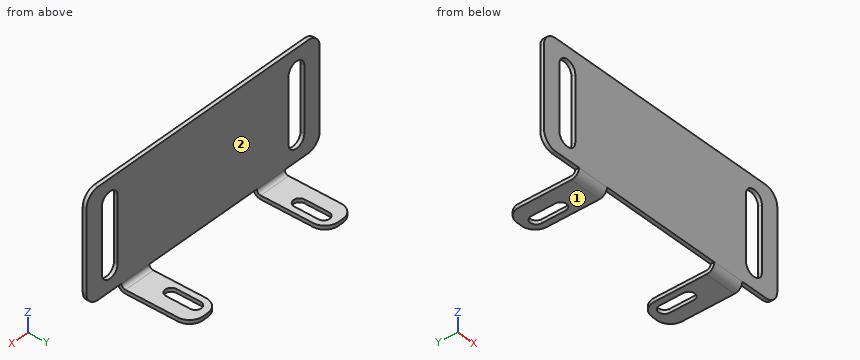
```python
from build123d import *

# Parameters (mm, degrees)
SKETCH1_W             = 50
SKETCH1_H             = 20
BASE_FLANGE1_DEPTH    = 0.7
EDGE_FLANGE1_DEPTH    = 6
CUT_EXTRUDE1_REACH    = 37.405
BREAK_CORNER1_START   = -12
BREAK_CORNER1_DEPTH   = 2
BREAK_CORNER1_START_2 = -2
BREAK_CORNER1_2_DEPTH = 3
CUT_EXTRUDE2_REACH    = 32.41


with BuildPart() as part:
    # Base-Flange1: sheet metal written as solids
    # Sketch1 → Base-Flange1 (new body)
    with BuildSketch(Plane(origin=(0, 0, 0), x_dir=(1, 0, 0), z_dir=(0, 1, 0))):
        Rectangle(SKETCH1_W, SKETCH1_H)
    extrude(amount=-BASE_FLANGE1_DEPTH)

    # Edge-Flange1: sheet metal written as solids
    # Edge-Flange1 section (on a plane across the edge) → Edge-Flange1 (add)
    with BuildSketch(Plane(origin=(17.5, 0, -10.7366), x_dir=(0, 0, 1), z_dir=(-1, 0, 0))):
        with BuildLine():
            Line((-0.7, 0.7366), (-0.7, 13))
            Line((-0.7, 13), (0, 13))
            Line((0, 13), (0, 0.7366))
            ThreePointArc((0, 0.7366), (0.215745145, 0.215745145), (0.7366, 0))
            Line((0.7366, 0), (0.7366, -0.7))
            ThreePointArc((0.7366, -0.7), (-0.279229602, -0.279229602), (-0.7, 0.7366))
        make_face()
    edge_flange1 = extrude(amount=EDGE_FLANGE1_DEPTH)

    # Sketch7 → Cut-Extrude1 (cut, up to next)
    with BuildSketch(Plane(origin=(0, 0, -11.4366), x_dir=(-1, 0, 0), z_dir=(0, 0, -1)), mode=Mode.PRIVATE) as cut_extrude1_sk1:
        with BuildLine():
            Line((-12.65, 10.5), (-12.65, 6))
            ThreePointArc((-12.65, 6), (-13.75, 4.9), (-14.85, 6))
            Line((-14.85, 6), (-14.85, 10.5))
            ThreePointArc((-14.85, 10.5), (-13.75, 11.6), (-12.65, 10.5))
        make_face()
    cut_extrude1_tool1 = extrude(cut_extrude1_sk1.sketch, amount=-CUT_EXTRUDE1_REACH, mode=Mode.PRIVATE) & part.part
    cut_extrude1 = cut_extrude1_tool1.solids().sort_by_distance((13.75, 8.25, -11.4366))[0]
    add(cut_extrude1, mode=Mode.SUBTRACT)

    # Mirror1: Edge-Flange1, Cut-Extrude1 across plane
    add(edge_flange1.mirror(Plane(origin=(0, 0, 0), x_dir=(0, 0, 1), z_dir=(1, 0, 0))))
    add(cut_extrude1.mirror(Plane(origin=(0, 0, 0), x_dir=(0, 0, 1), z_dir=(1, 0, 0))), mode=Mode.SUBTRACT)

    # Break-Corner1: read off the stored shape, not the designer's step
    # Break-Corner1 outline → Break-Corner1 (cut)
    with BuildSketch(Plane.XY.offset(BREAK_CORNER1_START)):
        with BuildLine():
            ThreePointArc((-17.5, 10.5), (-16.767766953, 12.267766953), (-15, 13))
            Line((-15, 13), (-17.5, 13))
            Line((-17.5, 13), (-17.5, 10.5))
        make_face()
        with BuildLine():
            ThreePointArc((-14, 13), (-12.232233047, 12.267766953), (-11.5, 10.5))
            Line((-11.5, 10.5), (-11.5, 13))
            Line((-11.5, 13), (-14, 13))
        make_face()
        with BuildLine():
            ThreePointArc((11.5, 10.5), (12.232233047, 12.267766953), (14, 13))
            Line((14, 13), (11.5, 13))
            Line((11.5, 13), (11.5, 10.5))
        make_face()
        with BuildLine():
            ThreePointArc((15, 13), (16.767766953, 12.267766953), (17.5, 10.5))
            Line((17.5, 10.5), (17.5, 13))
            Line((17.5, 13), (15, 13))
        make_face()
    extrude(amount=BREAK_CORNER1_DEPTH, mode=Mode.SUBTRACT)

    # Break-Corner1 2 outline → Break-Corner1 2 (cut)
    with BuildSketch(Plane(origin=(0, 0, 0), x_dir=(1, 0, 0), z_dir=(0, 1, 0)).offset(BREAK_CORNER1_START_2)):
        with BuildLine():
            ThreePointArc((22.5, 10), (24.267766953, 9.267766953), (25, 7.5))
            Line((25, 7.5), (25, 10))
            Line((25, 10), (22.5, 10))
        make_face()
        with BuildLine():
            Line((-25, 10), (-25, 7.5))
            ThreePointArc((-25, 7.5), (-24.267766953, 9.267766953), (-22.5, 10))
            Line((-22.5, 10), (-25, 10))
        make_face()
        with BuildLine():
            Line((-25, -10), (-22.5, -10))
            ThreePointArc((-22.5, -10), (-24.267766953, -9.267766953), (-25, -7.5))
            Line((-25, -7.5), (-25, -10))
        make_face()
        with BuildLine():
            ThreePointArc((25, -7.5), (24.267766953, -9.267766953), (22.5, -10))
            Line((22.5, -10), (25, -10))
            Line((25, -10), (25, -7.5))
        make_face()
    extrude(amount=BREAK_CORNER1_2_DEPTH, mode=Mode.SUBTRACT)

    # Sketch8 → Cut-Extrude2 (cut, up to next)
    with BuildSketch(Plane(origin=(0, 0, 0), x_dir=(1, 0, 0), z_dir=(0, 1, 0)), mode=Mode.PRIVATE) as cut_extrude2_sk1:
        with BuildLine():
            Line((-18.3, 6), (-18.3, -6))
            ThreePointArc((-18.3, -6), (-20, -7.7), (-21.7, -6))
            Line((-21.7, -6), (-21.7, 6))
            ThreePointArc((-21.7, 6), (-20, 7.7), (-18.3, 6))
        make_face()
    cut_extrude2_tool1 = extrude(cut_extrude2_sk1.sketch, amount=-CUT_EXTRUDE2_REACH, mode=Mode.PRIVATE) & part.part
    # Sketch8 → Cut-Extrude2 (cut, up to next)
    with BuildSketch(Plane(origin=(0, 0, 0), x_dir=(1, 0, 0), z_dir=(0, 1, 0)), mode=Mode.PRIVATE) as cut_extrude2_sk2:
        with BuildLine():
            Line((18.3, 6), (18.3, -6))
            ThreePointArc((18.3, -6), (20, -7.7), (21.7, -6))
            Line((21.7, -6), (21.7, 6))
            ThreePointArc((21.7, 6), (20, 7.7), (18.3, 6))
        make_face()
    cut_extrude2_tool2 = extrude(cut_extrude2_sk2.sketch, amount=-CUT_EXTRUDE2_REACH, mode=Mode.PRIVATE) & part.part
    add(cut_extrude2_tool1.solids().sort_by_distance((-20, 0, 0))[0], mode=Mode.SUBTRACT)
    add(cut_extrude2_tool2.solids().sort_by_distance((20, 0, 0))[0], mode=Mode.SUBTRACT)


solid = part.part
```
Source: CAD feature listing. Evaluate the final solid. Frame: model axes, mm. Face numbers are marked on the shaded views. A direction names the side the tool comes from. Give positions to 0.01 mm unless a question says otherwise; leave off trailing zeros. Write each loop counter-clockwise with the first axis right and the second up, starting at its lowest first coordinate (ties: lowest second). Pieces come first, ordered by that corner, then holes. Notation, with made-up numbers: (16.5, 81.25) - (37.5, 81.25) arc R11 ccw to (37.5, 92.25) - close; hole circle Ø6 at (-21.75, 58.25). An arc over 180 degrees is marked (long way). One line per item, written item: value. Start each with the question number.
Q1. First-contact query: pin 1 Ø1.5 at (x, z) = (-20, -2) entering from -Y; pin 2 Ø0.6 at (y, z) = (8.5, -11) entering from -X; pin 3 Ø1.8 at (x, y) = (14.5, 5) entering from +Z; pin 4 Ø0.6 at (x, y) = (21, -0.5) entering from -Z. Flat tips, straight axial feed; report the tip coordinate or a pass-through.
Q2. Section query C-C, the plane x = -20. Return the cut outline in (y, z), then the cut area to 3 significant figures.
Q3. Section query B-B, the plane y = 8.75. Return the cut outline in (x, z).
Q4. Material intervals for probe 1 along Y at (x, z) = (8, 1); probe 2 along Z at (x, y) = (17, 5), sorted ascending. Write a range as from..to.
Q5. Section query D-D, the plane x = -1.5. Return the cut outline in (y, z).
Q6. Section query A-A, the plane z = 0.5. Return the cut outline in (x, y), then the cut area to 3 significant figures.
Q7. Set-up query: the marked faces 1 and 2. Return all of +Z, -Z, +X, -X, +Y, -Y with unobstructed straight access to the full face (end or side cutting, diameter ignored); none if empty.
Answer:
1. pin 1: passes through
1. pin 2: stops at x = -17.5
1. pin 3: stops at z = -10.74
1. pin 4: stops at z = -10
2. outline: (-0.7, -10) - (0, -10) - (0, -7.7) - (-0.7, -7.7) - close; (-0.7, 7.7) - (0, 7.7) - (0, 10) - (-0.7, 10) - close
2. area: 3.22 mm2
3. outline: (-17.5, -11.44) - (-14.85, -11.44) - (-14.85, -10.74) - (-17.5, -10.74) - close; (-12.65, -11.44) - (-11.5, -11.44) - (-11.5, -10.74) - (-12.65, -10.74) - close; (11.5, -11.44) - (12.65, -11.44) - (12.65, -10.74) - (11.5, -10.74) - close; (14.85, -11.44) - (17.5, -11.44) - (17.5, -10.74) - (14.85, -10.74) - close
4. probe 1: y = -0.7..0
4. probe 2: z = -11.44..-10.74
5. outline: (-0.7, -10) - (0, -10) - (0, 10) - (-0.7, 10) - close
6. outline: (-25, -0.7) - (-21.7, -0.7) - (-21.7, 0) - (-25, 0) - close; (-18.3, -0.7) - (18.3, -0.7) - (18.3, 0) - (-18.3, 0) - close; (21.7, -0.7) - (25, -0.7) - (25, 0) - (21.7, 0) - close
6. area: 30.2 mm2
7. face 1: -Z, +X, -X, +Y, -Y
7. face 2: +Z, +X, -X, +Y
